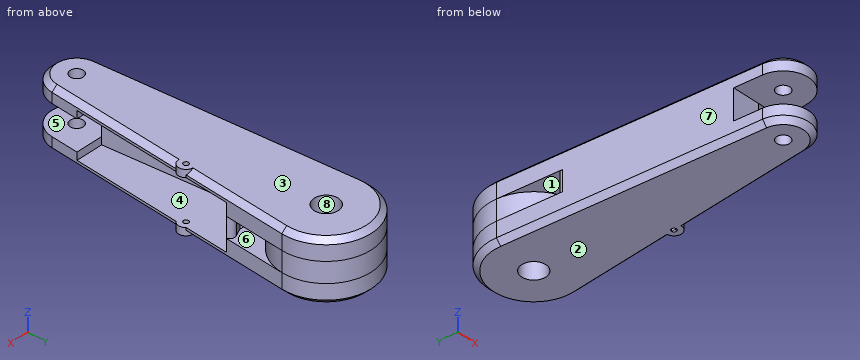
```python
from build123d import *

# Parameters (mm, degrees)
SKETCH1_R                = 45
SKETCH1_R_2              = 12
BOSS_EXTRUDE1_DEPTH      = 30
SKETCH2_R                = 6.500000000000002
BOSS_EXTRUDE2_DEPTH      = 60.00000000000001
CUT_EXTRUDE1_DEPTH       = 15
CHAMFER1_SIZE            = 5
SKETCH4_R                = 68.57027417716169
CUT_EXTRUDE3_DEPTH       = 10
FILLET1_R                = 5
CUT_EXTRUDE4_DEPTH       = 281.26772914483035
CUT_EXTRUDE4_DEPTH_BACK  = 281.26772914483035
SKETCH5_R                = 2.5000000000000058
BOSS_EXTRUDE3_DEPTH      = 30
BOSS_EXTRUDE3_DEPTH_BACK = 30
SKETCH6_R                = 7.499999999999997
SKETCH6_R_2              = 2.5000000000000058
CUT_EXTRUDE5_DEPTH       = 22.5


with BuildPart() as part:
    # Sketch1 → Boss-Extrude1 (new, symmetric)
    with BuildSketch(Plane.XY):
        Circle(SKETCH1_R)
        Circle(SKETCH1_R_2, mode=Mode.SUBTRACT)
    extrude(amount=BOSS_EXTRUDE1_DEPTH, both=True)

    # Sketch2 → Boss-Extrude2 (add)
    with BuildSketch(Plane.XY.offset(30)):
        with BuildLine():
            Line((-44.85576885975762, -3.600000000000007), (-24.91987158875419, -252))
            ThreePointArc((-24.91987158875419, -252), (3.215e-14, -275), (24.91987158875426, -252))
            Line((24.91987158875426, -252), (44.85576885975761, -3.5999999999999956))
            ThreePointArc((44.85576885975761, -3.5999999999999956), (2.76e-15, -45.000000000000014), (-44.85576885975762, -3.600000000000007))
        make_face()
        with Locations((3.062e-14, -250)):
            Circle(SKETCH2_R, mode=Mode.SUBTRACT)
    extrude(amount=-BOSS_EXTRUDE2_DEPTH)

    # Sketch3 → Cut-Extrude1 (cut, symmetric)
    with BuildSketch(Plane.XY):
        with BuildLine():
            Line((-27.08681694429805, -225), (-24.91987158875419, -252))
            ThreePointArc((-24.91987158875419, -252), (3.215e-14, -275), (24.91987158875426, -252))
            Line((24.91987158875426, -252), (27.086816944298096, -225))
            Line((27.086816944298096, -225), (-27.08681694429805, -225))
        make_face()
    extrude(amount=CUT_EXTRUDE1_DEPTH, both=True, mode=Mode.SUBTRACT)

    # Chamfer1
    chamfer1_edges = [part.edges().sort_by_distance(p)[0] for p in [
        (-1.599e-14, 44.99999999999999, 30),
        (5.77e-15, 44.99999999999999, -29.99999999999991),
        (34.88782022425593, -127.8, -30.000000000000007),
        (3.042e-14, -275, -30.000000000000007),
        (-34.887820224255904, -127.80000000000001, -30.000000000000007),
        (-34.887820224255904, -127.80000000000001, 30),
        (3.042e-14, -275, 30),
        (34.88782022425593, -127.8, 30),
    ]]
    chamfer(chamfer1_edges, length=CHAMFER1_SIZE)

    # Sketch4 → Cut-Extrude3 (cut, symmetric)
    with BuildSketch(Plane.XY):
        Circle(SKETCH4_R)
        with BuildLine():
            ThreePointArc((44.99999999999999, 4.4e-16), (44.963927757087085, -1.8014440472726034), (44.8557688597576, -3.599999999999995))
            ThreePointArc((44.855768859757625, -3.600000000000005), (-8.27e-15, -45.00000000000002), (-44.855768859757625, -3.6000000000000085))
            ThreePointArc((-44.85576885975762, -3.6000000000000054), (-1.8014440472726134, 44.963927757087085), (44.99999999999999, 4.4e-16))
        make_face(mode=Mode.SUBTRACT)
    extrude(amount=CUT_EXTRUDE3_DEPTH, both=True, mode=Mode.SUBTRACT)

    # Fillet1
    # the kernel refuses this fillet: 5 mm, written as the material it takes off along each edge
    with BuildSketch(Plane(origin=(-40.716681036978386, -55.17276851911722, -10), x_dir=(0.07999999999999997, -0.9967948635501691, 0), z_dir=(0, 0, 1))) as fillet1_piece_1:
        with BuildLine():
            CenterArc((10.007537661154231, 4.999999999999998), FILLET1_R, 147.0642758003335, 122.9357241996666)
            ThreePointArc((5.81113251406956, 7.7184892572017425), (3.041676337682726, 3.7567694305680726), (0, 0))
            Line((0, 0), (10.007537661154236, 2e-17))
        make_face()
    extrude(amount=20, mode=Mode.SUBTRACT)
    with BuildSketch(Plane(origin=(40.7166810369784, -55.17276851911721, -10), x_dir=(-0.08000000000000003, -0.9967948635501691, 0), z_dir=(0, 0, 1))) as fillet1_piece_2:
        with BuildLine():
            CenterArc((10.007537661154224, -4.999999999999998), FILLET1_R, 89.99999999999993, 122.93572419966637)
            ThreePointArc((5.811132514069545, -7.718489257201729), (3.0416763376827105, -3.756769430568052), (0, 0))
            Line((0, 0), (10.00753766115423, -4e-17))
        make_face()
    extrude(amount=20, mode=Mode.SUBTRACT)

    # Sketch5 → Cut-Extrude4 (cut, two sides: drawn at the far end of the back side and taken through both)
    with BuildSketch(Plane.XY.offset(-CUT_EXTRUDE4_DEPTH_BACK)):
        with Locations(Location((31.135897271003447, -112.0487191029763, 0), (0, 0, 85.411434264))):
            Circle(SKETCH5_R)
    extrude(amount=CUT_EXTRUDE4_DEPTH + CUT_EXTRUDE4_DEPTH_BACK, mode=Mode.SUBTRACT)

    # Sketch6 → Boss-Extrude3 (add, two sides: drawn at the far end of the back side and taken through both)
    with BuildSketch(Plane.XY.offset(-BOSS_EXTRUDE3_DEPTH_BACK)):
        with Locations((31.135897271003447, -112.0487191029763)):
            Circle(SKETCH6_R)
        with Locations((31.135897271003447, -112.0487191029763)):
            Circle(SKETCH6_R_2, mode=Mode.SUBTRACT)
    extrude(amount=BOSS_EXTRUDE3_DEPTH + BOSS_EXTRUDE3_DEPTH_BACK)

    # Sketch8 → Cut-Extrude5 (cut, symmetric)
    with BuildSketch(Plane.XY):
        Polygon((39.65576885975762, -225), (39.655768859757615, -68.39166613076095), (40.05576885975761, -63.40769181301013), (0, -65.20900375479165), (-13.97990070496815, -65.20900375479165), (2.082e-14, -225), (27.086816944298096, -225), align=None)
    extrude(amount=CUT_EXTRUDE5_DEPTH, both=True, mode=Mode.SUBTRACT)


solid = part.part
```
Design review of the part built by this model. Coordinates are the model's own, in mm. Face numbers are marked on the shaded views. A direction names the side the tool comes from. Give positions to 0.01 mm unless a question says otherwise; leave off trailing zeros. Write each loop counter-clockwise with the first axis right and the second up, starting at its lowest first coordinate (ties: lowest second). Pieces come first, ordered by that corner, then holes. Notation, with made-up numbers: (44, 48.5) -> (89, 48.5) arc R21 cw to (89, 82.5) -> close; hole circle Ø8 at (-25.5, -38). An arc over 180 degrees is marked (long way). Answer in a Markdown table with one row per item.
(1) Clearance check with flat-ended pins moving along their axes: pin 1 (4 mm diameter, centred on x = -3.5, z = -16, fed in from -Y); pin 2 (5 mm diameter, centred on x = 3.5, z = -15.5, fed in from +Y); pin 3 (21.5 mm diameter, centred on x = -14, z = 4.5, fed in from -Y); pin 4 (8 mm diameter, centred on x = 0, y = -250, fed in from +Z). State where each tip first meets the part, or that it passes through.
Results:
| item | result |
|---|---|
| pin 1 | y = -274.95 |
| pin 2 | y = 44.99 |
| pin 3 | y = -272.1 |
| pin 4 | through |
(2) For the marked faces 4, 5, 6, 7 and 8, list the 3-axis set-ups (+Z, -Z, +X, -X, +Y, -Y) from which the entire face can be reached by the end or side of a thin tool; tool diameter is ignored.
Results:
| item | result |
|---|---|
| face 4 | +X |
| face 5 | +X, -X, -Y |
| face 6 | none |
| face 7 | +Z, -Z, -X, -Y |
| face 8 | +Z, -Z |
(3) Consider section A-A (z = 2). State the section outline as (x, y) points, then the cut area to 3 significant figures.
Results:
| item | result |
|---|---|
| outline | circle Ø90 at (0, 0); (-39.92, -65.15) -> (-27.09, -225) -> (0, -225) -> (-13.81, -67.17) arc R68.57 cw to (-32.56, -60.35) arc R5 ccw to start; (24.31, -64.12) -> (39.75, -63.42) arc R5 ccw to (32.56, -60.35) arc R68.57 cw to start; hole circle Ø24 at (0, 0) |
| area | 10,200 mm2 |
(4) Mouldability with a two-part tool opening along Z and no side actions: class the marked faces 1, 2 and 3 as +Z half, -Z half, draft (parallel to the pull), parting line (faces both ways), or undercut.
Results:
| item | result |
|---|---|
| face 1 | undercut |
| face 2 | -Z half |
| face 3 | +Z half |
(5) To check wall thickness, follow probe 1 along Z at (x, y) = (17.5, -138); probe 2 along Z at (x, y) = (10, -248); probe 3 along Y at (x, z) = (-19.5, -5). State the ranges of each line that lie inside material, in increasing order.
Results:
| item | result |
|---|---|
| probe 1 | -30 to -22.5, 22.5 to 30 |
| probe 2 | -30 to -15, 15 to 30 |
| probe 3 | -225 to -65.74, -40.56 to 40.56 |
(6) Consider section B-B (y = 0). State the section outline as (x, z) points.
Results:
| item | result |
|---|---|
| outline | (-45, -25) -> (-40, -30) -> (-12, -30) -> (-12, 30) -> (-40, 30) -> (-45, 25) -> close; (12, -30) -> (40, -30) -> (45, -25) -> (45, 25) -> (40, 30) -> (12, 30) -> close |
